For this review, take the finished solid that the model builds, in its own axes (mm). Face numbers are marked on the shaded views. A direction names the side the tool comes from. Coordinates: 2 decimals unless noted, no trailing zeros. Loops run counter-clockwise (first coordinate to the right, second up) from the corner with the lowest first, then second, coordinate; pieces in that order, holes last. Notation, with made-up numbers: (19.25, 88) - (37.25, 88) arc R29 ccw to (37.25, 114) - close; hole circle Ø10 at (30, -31.5). An arc over 180 degrees is marked (long way). Answer as a JSON object with one key per item and string values. Group by question number.
Item 1: We need section D-D (y = 17). Give the boundary of the cut face in (x, z).
Item 2: To check wall thickness, follow line 1 (Y direction, x = 55, z = 1.75); line 2 (Y direction, x = 75, z = 6.25); line 3 (Y direction, x = 79, z = 1). State the ranges of each line that lie inside material, in increasing order.
Item 3: We need section A-A (z = 4). Give the boundary of the cut face in (x, y) (3 decimals), then the cut area to 3 significant figures.
Item 4: We need section C-C (y = 92). Give the boundary of the cut face in (x, z).
Item 5: Clearance check with flat-ended pins moving along their axes: pin 1 (1 mm diameter, centred on x = 45, z = 6.5, fed in from +Y); pin 2 (3 mm diameter, centred on y = 50.5, z = 1, fed in from -X); pin 3 (1.8 mm diameter, centred on x = 55.5, z = 6.5, fed in from -Y). State where each tip first meets the part, or that it passes through.
Item 6: We need section B-B (x = 89). Give the boundary of the cut face in (y, z), then the cut area to 3 significant figures.
Item 7: Tool access review of the marked faces 1 and 2: name each direction out of +Z, -Z, +X, -X, +Y, -Y from which nothing blocks a thin tool from reaching the whole face with its end or side.
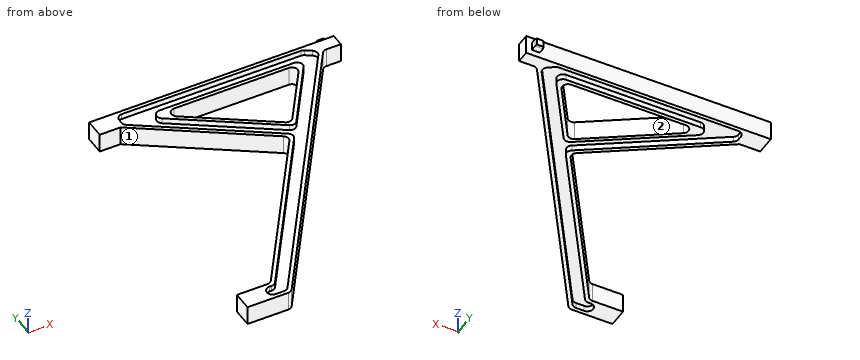
from build123d import *

# Parameters (mm, degrees)
F1_DEPTH    = 1.5875
F0_W        = 3.175
F0_H        = 3.81
F2_DEPTH    = 3.81
F0_H_2      = 3.175
F3_DEPTH    = 1.5875
F5_R        = 2.28599
F6_C1_SIZE2 = 0.254
F6_C1_SIZE  = 0.762
F6_C2_SIZE2 = 0.254
F6_C2_SIZE  = 0.762
F6_C3_SIZE2 = 0.762
F6_C3_SIZE  = 0.254
F6_C4_SIZE2 = 0.762
F6_C4_SIZE  = 0.254


# Not quite as in the source:
# - a fillet or chamfer is up to 0.001 mm smaller than in the source, because OpenCascade refuses the exact size


with BuildPart() as f1:
    # F0 (on Top) → F1 (new body, symmetric)
    with BuildSketch(Plane.XY):
        Polygon((84.7879795397, 75.6059451024), (107.4843514416, 109.6505029552), (102.7961058745, 112.776), (28.5815359464, 112.776), (28.5815359464, 107.4966776252), (78.4441827097, 74.332540073), (32.9531559943, 6.096), (28.5815359464, 6.096), (28.5815359464, 1.524), (35.4000161381, 1.524), (82.2518902426, 71.8018111567), align=None)
        Polygon((35.7737204145, 108.204), (101.0251559943, 108.204), (80.9802734819, 78.1366762315), align=None, mode=Mode.SUBTRACT)
    extrude(amount=F1_DEPTH, both=True)

    # F0 (on Top) → F2 (join, symmetric)
    with BuildSketch(Plane.XY):
        Polygon((27.0575359464, 3.81), (27.0575359464, 0), (36.215636186, 0), (109.0289695194, 109.22), (115.9575359464, 109.22), (115.9575359464, 114.3), (113.7350359464, 114.3), (110.5600359464, 114.3), (103.2575359464, 114.3), (27.0575359464, 114.3), (18.8025359464, 114.3), (18.8025359464, 106.68), (23.8825359464, 106.68), (23.8825359464, 110.49), (27.0575359464, 110.49), (27.0575359464, 106.68), (76.2944590233, 73.8553846154), (32.1375359464, 7.62), (27.0575359464, 7.62), (18.8025359464, 7.62), (18.8025359464, 0), (23.8825359464, 0), (23.8825359464, 3.81), align=None)
        Polygon((102.7961058745, 112.776), (107.4843514416, 109.6505029552), (84.7879795397, 75.6059451024), (82.2518902426, 71.8018111567), (35.4000161381, 1.524), (28.5815359464, 1.524), (28.5815359464, 6.096), (32.9531559943, 6.096), (78.4441827097, 74.332540073), (28.5815359464, 107.4966776252), (28.5815359464, 112.776), align=None, mode=Mode.SUBTRACT)
        Polygon((80.9802734819, 78.1366762315), (101.0251559943, 108.204), (35.7737204145, 108.204), align=None)
        Polygon((80.5212745185, 80.1956078582), (40.7946863059, 106.68), (98.1775359464, 106.68), align=None, mode=Mode.SUBTRACT)
        with Locations((25.4700359464, 1.905)):
            Rectangle(F0_W, F0_H)
        with Locations((25.4700359464, 108.585)):
            Rectangle(F0_W, F0_H)
    extrude(amount=F2_DEPTH, both=True)

    # F0 (on Top) → F3 (join, symmetric)
    with BuildSketch(Plane.XY):
        with Locations((112.1475359464, 115.8875)):
            Rectangle(F0_W, F0_H_2)
    extrude(amount=F3_DEPTH, both=True)


with BuildPart() as f1_1:
    # F4: moved
    add(f1.part.moved(Location((0, 0, 3.81))))

    # F5 (radius 2.286 in the source; OpenCascade refuses exactly that, so slightly less here)
    f5_edges = [f1_1.edges().sort_by_distance(p)[0] for p in [
        (35.77372, 108.204, 6.50875),
        (35.77372, 108.204, 1.11125),
        (101.025156, 108.204, 6.50875),
        (101.025156, 108.204, 1.11125),
        (80.980273, 78.136676, 1.11125),
        (80.980273, 78.136676, 6.50875),
        (78.444183, 74.33254, 6.50875),
        (78.444183, 74.33254, 1.11125),
        (102.796106, 112.776, 6.50875),
        (102.796106, 112.776, 1.11125),
        (28.581536, 112.776, 6.50875),
        (28.581536, 107.496678, 6.50875),
        (28.581536, 107.496678, 1.11125),
        (28.581536, 112.776, 1.11125),
        (32.953156, 6.096, 6.50875),
        (32.953156, 6.096, 1.11125),
        (35.400016, 1.524, 1.11125),
        (35.400016, 1.524, 6.50875),
        (28.581536, 6.096, 6.50875),
        (28.581536, 1.524, 6.50875),
        (28.581536, 1.524, 1.11125),
        (28.581536, 6.096, 1.11125),
        (107.484351, 109.650503, 6.50875),
        (107.484351, 109.650503, 1.11125),
        (109.02897, 109.22, 3.81),
        (36.215636, 0, 3.81),
        (76.294459, 73.855385, 3.81),
        (32.137536, 7.62, 3.81),
        (40.794686, 106.68, 3.81),
        (80.521275, 80.195608, 3.81),
        (98.177536, 106.68, 3.81),
    ]]
    fillet(f5_edges, radius=F5_R)

    # F6: chamfer of 0.254 x 0.762 on 4 edges, made by hand

    # F6_c1
    f6_c1_edges = [f1_1.edges().sort_by_distance(p)[0] for p in [
        (110.5600359464, 117.475, 3.81),
    ]]
    f6_c1_side = f1_1.faces().sort_by_distance((110.5600359464, 117.46992, 3.81))[0]
    chamfer(f6_c1_edges, length=F6_C1_SIZE, length2=F6_C1_SIZE2, reference=f6_c1_side)

    # F6_c2
    f6_c2_edges = [f1_1.edges().sort_by_distance(p)[0] for p in [
        (112.2745359464, 117.475, 5.3975),
    ]]
    f6_c2_side = f1_1.faces().sort_by_distance((112.2745359464, 117.46992, 5.3975))[0]
    chamfer(f6_c2_edges, length=F6_C2_SIZE, length2=F6_C2_SIZE2, reference=f6_c2_side)

    # F6_c3
    f6_c3_edges = [f1_1.edges().sort_by_distance(p)[0] for p in [
        (113.7350359464, 117.475, 3.683),
    ]]
    f6_c3_side = f1_1.faces().sort_by_distance((113.7299559464, 117.475, 3.683))[0]
    chamfer(f6_c3_edges, length=F6_C3_SIZE, length2=F6_C3_SIZE2, reference=f6_c3_side)

    # F6_c4
    f6_c4_edges = [f1_1.edges().sort_by_distance(p)[0] for p in [
        (112.1475359464, 117.475, 2.2225),
    ]]
    f6_c4_side = f1_1.faces().sort_by_distance((112.1475359464, 117.475, 2.22758))[0]
    chamfer(f6_c4_edges, length=F6_C4_SIZE, length2=F6_C4_SIZE2, reference=f6_c4_side)


solid = f1_1.part
Check sheet entries:
{
 "1": {"outline": "(38.39, 0) - (40.22, 0) - (40.22, 2.22) - (45.72, 2.22) - (45.72, 0) - (47.55, 0) - (47.55, 7.62) - (45.72, 7.62) - (45.72, 5.4) - (40.22, 5.4) - (40.22, 7.62) - (38.39, 7.62) - close"},
 "2": {"line 1": "y = 28.18 to 30.92, 39.17 to 41.91, 88.05 to 89.93, 95.42 to 97.21, 106.68 to 108.2, 112.78 to 114.3", "line 2": "y = 58.18 to 60.92, 69.17 to 71.91, 74.53 to 76.62, 82.11 to 83.88, 106.68 to 108.2, 112.78 to 114.3", "line 3": "y = 64.18 to 66.92, 79.45 to 81.26, 106.68 to 108.2, 112.78 to 114.3"},
 "3": {"outline": "(18.803, 0) - (34.992, 0) arc R2.286 ccw to (36.894, 1.018) - (108.35, 108.202) arc R2.286 cw to (110.252, 109.22) - (115.958, 109.22) - (115.958, 114.3) - (113.735, 114.3) - (113.735, 116.713) - (113.481, 117.475) - (110.814, 117.475) - (110.56, 116.713) - (110.56, 114.3) - (18.803, 114.3) - (18.803, 106.68) - (27.058, 106.68) - (74.392, 75.123) arc R2.286 cw to (75.026, 71.953) - (32.816, 8.638) arc R2.286 cw to (30.914, 7.62) - (18.803, 7.62) - close; hole (47.077, 102.492) - (78.619, 81.464) arc R2.286 ccw to (81.789, 82.098) - (95.808, 103.126) arc R2.286 ccw to (93.906, 106.68) - (48.345, 106.68) arc R2.286 ccw to start", "area": "2,210 mm2"},
 "4": {"outline": "(49.08, 0) - (51.88, 0) - (51.88, 2.22) - (60.14, 2.22) - (60.14, 0) - (62.81, 0) - (62.81, 7.62) - (60.14, 7.62) - (60.14, 5.4) - (51.88, 5.4) - (51.88, 7.62) - (49.08, 7.62) - close; (88.39, 0) - (90.22, 0) - (90.22, 2.22) - (95.72, 2.22) - (95.72, 0) - (97.55, 0) - (97.55, 7.62) - (95.72, 7.62) - (95.72, 5.4) - (90.22, 5.4) - (90.22, 7.62) - (88.39, 7.62) - close"},
 "5": {"pin 1": "stops at y = 114.3", "pin 2": "stops at x = 59.72", "pin 3": "stops at y = 27.58"},
 "6": {"outline": "(79.18, 0) - (81.92, 0) - (81.92, 2.22) - (90.17, 2.22) - (90.17, 0) - (92.91, 0) - (92.91, 7.62) - (90.17, 7.62) - (90.17, 5.4) - (81.92, 5.4) - (81.92, 7.62) - (79.18, 7.62) - close; (106.68, 0) - (108.2, 0) - (108.2, 2.22) - (112.78, 2.22) - (112.78, 0) - (114.3, 0) - (114.3, 7.62) - (112.78, 7.62) - (112.78, 5.4) - (108.2, 5.4) - (108.2, 7.62) - (106.68, 7.62) - close", "area": "106 mm2"},
 "7": {"face 1": "+Z, -Z, -X", "face 2": "+Z, -Z"}
}
